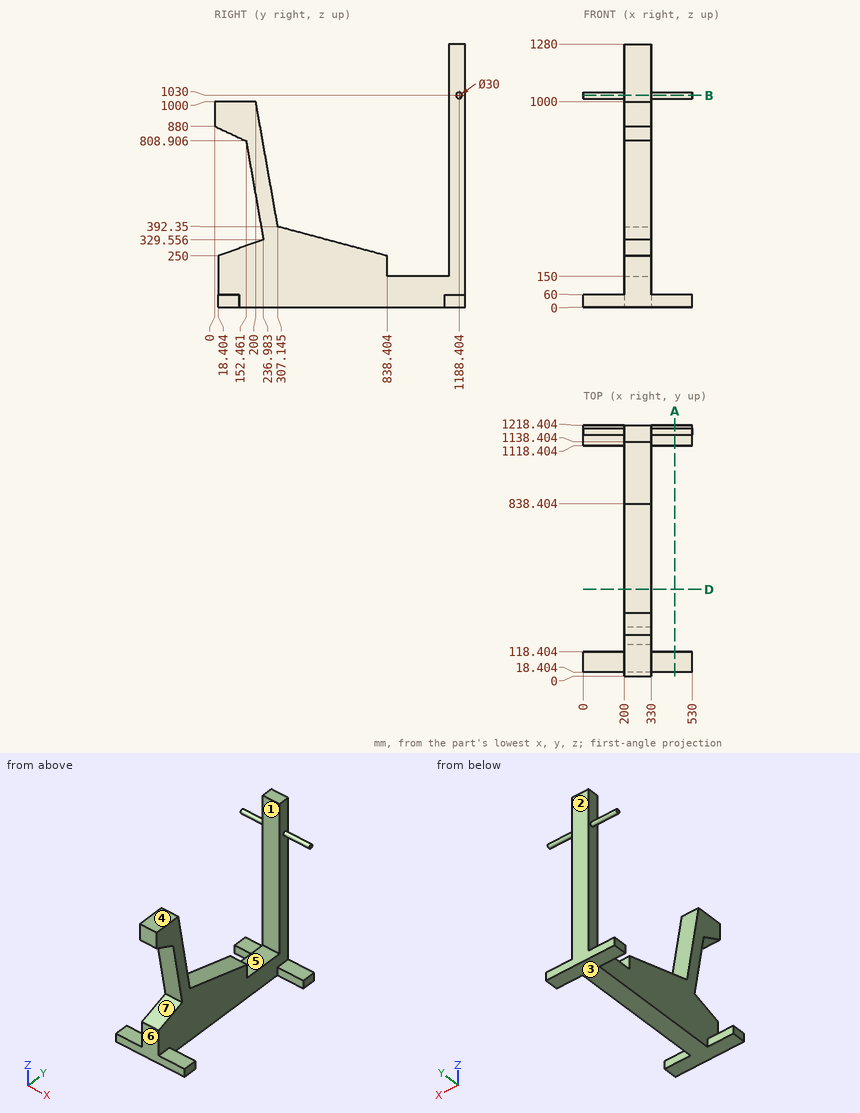
Check sheet for the drawn part. Datum: minimum x, y, z corner. Units: mm. A direction names the side the tool comes from. Coordinates: 2 decimals unless noted, no trailing zeros. Loops run counter-clockwise (first coordinate to the right, second up) from the corner with the lowest first, then second, coordinate; pieces in that order, holes last. Notation, with made-up numbers: (31.25, 24) -> (41.25, 24) arc R27 cw to (41.25, 56) -> close; hole circle Ø5 at (51, -37.5). An arc over 180 degrees is marked (long way). Answer as a JSON object with one key per item and string values. Group by question number.
Item 1: Scan lines: probe 1 along X at (y, z) = (260.5, 279.5); probe 2 along Z at (x, y) = (221.5, 1032); probe 3 along Z at (x, y) = (220.5, 93.5). Record each from-to range of solid material in increasing order.
Item 2: Depth check by flat-ended pin: pin 1 (8 mm diameter, centred on y = 731.5, z = 171.5, fed in from -X). Enter the tip coordinate at first touch or a pass-through.
Item 3: Sectioned sample at A-A on x = 445.5. Record the boundary of the cut face in (y, z) (1 decimal).
Item 4: Mould release check, pull along Y, two halves, no side actions. Record for the marked faces 1, 2 and 3: +Y half, -Y half, draft (parallel to the pull), parting line (faces both ways), or undercut.
Item 5: Sectioned sample at D-D on y = 421.5. Record the boundary of the cut face in (x, z), plus the area to 3 significant figures.
Item 6: Sectioned sample at B-B on z = 1030. Record the boundary of the cut face in (x, y) (1 decimal), plus the area to 3 significant figures.
Item 7: Tool access check on the marked faces 4, 5, 6 and 7. Record the directions out of +Z, -Z, +X, -X, +Y, -Y that give a thin tool (end or side, any length) a straight path to the whole face; none if there is none.
Evaluation:
{
 "1": {"probe 1": "x = 200 to 330", "probe 2": "z = 0 to 150", "probe 3": "z = 0 to 277.33, 836.4 to 1000"},
 "2": {"pin 1": "stops at x = 200"},
 "3": {"outline": "(18.4, 0) -> (118.4, 0) -> (118.4, 60) -> (18.4, 60) -> close; (1118.4, 0) -> (1218.4, 0) -> (1218.4, 60) -> (1118.4, 60) -> close; circle Ø30 at (1188.4, 1030)"},
 "4": {"face 1": "undercut", "face 2": "+Y half", "face 3": "draft"},
 "5": {"outline": "(200, 0) -> (330, 0) -> (330, 361.71) -> (200, 361.71) -> close", "area": "47,000 mm²"},
 "6": {"outline": "(0, 1173.4) -> (200, 1173.4) -> (200, 1138.4) -> (330, 1138.4) -> (330, 1173.4) -> (530, 1173.4) -> (530, 1203.4) -> (330, 1203.4) -> (330, 1218.4) -> (200, 1218.4) -> (200, 1203.4) -> (0, 1203.4) -> close", "area": "22,400 mm²"},
 "7": {"face 4": "+Z, +X, -X, -Y", "face 5": "+Z, +X, -X", "face 6": "-Z, +X, -X, -Y", "face 7": "+X, -X, -Y"}
}
